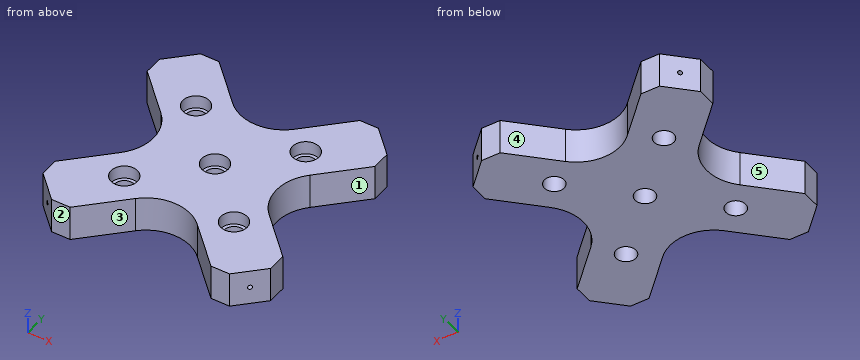
```python
from build123d import *

# Parameters (mm, degrees)
ESQUISSE1_R               = 2.25
BOSS_EXTRU_1_DEPTH        = 8
CONG_1_R                  = 10
ESQUISSE2_R               = 0.5
ENL_V_MAT_EXTRU_1_DEPTH   = 10
ESQUISSE3_R               = 3
ENL_V_MAT_EXTRU_2_DEPTH   = 3
SYM_TRIE2_COPY_1_SKETCH_R = 0.5
SYM_TRIE2_COPY_1_DEPTH    = 10
SYM_TRIE2_COPY_2_SKETCH_R = 3
SYM_TRIE2_COPY_2_DEPTH    = 3


with BuildPart() as part:
    # Esquisse1 → Boss.-Extru.1 (new body)
    with BuildSketch(Plane.XY):
        Polygon((-9.899494937, 0), (-25.935028843, 16.035533906), (-25.935028843, 20.278174593), (-20.278174593, 25.935028843), (-16.035533906, 25.935028843), (0, 9.899494937), (16.035533906, 25.935028843), (20.278174593, 25.935028843), (25.935028843, 20.278174593), (25.935028843, 16.035533906), (9.899494937, 0), (25.935028843, -16.035533906), (25.935028843, -20.278174593), (20.278174593, -25.935028843), (16.035533906, -25.935028843), (0, -9.899494937), (-16.035533906, -25.935028843), (-20.278174593, -25.935028843), (-25.935028843, -20.278174593), (-25.935028843, -16.035533906), align=None)
        with Locations((-12.5, -12.5)):
            Circle(ESQUISSE1_R, mode=Mode.SUBTRACT)
        with Locations((12.5, -12.5)):
            Circle(ESQUISSE1_R, mode=Mode.SUBTRACT)
        Circle(ESQUISSE1_R, mode=Mode.SUBTRACT)
        with Locations((12.5, 12.5)):
            Circle(ESQUISSE1_R, mode=Mode.SUBTRACT)
        with Locations((-12.5, 12.5)):
            Circle(ESQUISSE1_R, mode=Mode.SUBTRACT)
    extrude(amount=BOSS_EXTRU_1_DEPTH)

    # Congé1
    cong_1_edges = [part.edges().sort_by_distance(p)[0] for p in [
        (0, 9.899494937, 4),
        (9.899494937, 0, 4),
        (0, -9.899494937, 4),
        (-9.899494937, 0, 4),
    ]]
    fillet(cong_1_edges, radius=CONG_1_R)

    # Esquisse2 → Enlèv. mat.-Extru.1 (cut)
    with BuildSketch(Plane(origin=(23.106601718, 23.106601718, 0), x_dir=(0, 0, -1), z_dir=(0.707106781, 0.707106781, 0))):
        with Locations((-4, 0)):
            Circle(ESQUISSE2_R)
    enl_v_mat_extru_1 = extrude(amount=-ENL_V_MAT_EXTRU_1_DEPTH, mode=Mode.SUBTRACT)

    # Esquisse3 → Enlèv. mat.-Extru.2 (cut)
    with BuildSketch(Plane.XY.offset(8)):
        with Locations((12.5, 12.5)):
            Circle(ESQUISSE3_R)
        Circle(ESQUISSE3_R)
    enl_v_mat_extru_2 = extrude(amount=-ENL_V_MAT_EXTRU_2_DEPTH, mode=Mode.SUBTRACT)

    # Symétrie1: Enlèv. mat.-Extru.1, Enlèv. mat.-Extru.2 across plane
    add(enl_v_mat_extru_1.mirror(Plane.ZX), mode=Mode.SUBTRACT)
    add(enl_v_mat_extru_2.mirror(Plane.ZX), mode=Mode.SUBTRACT)

    # Symétrie2: Enlèv. mat.-Extru.1, Enlèv. mat.-Extru.2 across plane
    add(enl_v_mat_extru_1.mirror(Plane(origin=(0, 0, 0), x_dir=(0, 0, 1), z_dir=(1, 0, 0))), mode=Mode.SUBTRACT)
    add(enl_v_mat_extru_2.mirror(Plane(origin=(0, 0, 0), x_dir=(0, 0, 1), z_dir=(1, 0, 0))), mode=Mode.SUBTRACT)

    # Symétrie2 copy 1 sketch → Symétrie2 copy 1 (cut)
    with BuildSketch(Plane(origin=(-23.106601718, -23.106601718, 0), x_dir=(0, 0, -1), z_dir=(-0.707106781, -0.707106781, 0))):
        with Locations((-4, 0)):
            Circle(SYM_TRIE2_COPY_1_SKETCH_R)
    extrude(amount=-SYM_TRIE2_COPY_1_DEPTH, mode=Mode.SUBTRACT)

    # Symétrie2 copy 2 sketch → Symétrie2 copy 2 (cut)
    with BuildSketch(Plane(origin=(0, 0, 8), x_dir=(-1, 0, 0), z_dir=(0, 0, 1))):
        with Locations((12.5, 12.5)):
            Circle(SYM_TRIE2_COPY_2_SKETCH_R)
        Circle(SYM_TRIE2_COPY_2_SKETCH_R)
    extrude(amount=-SYM_TRIE2_COPY_2_DEPTH, mode=Mode.SUBTRACT)


solid = part.part
```
Geometry check sheet. Reference: the model listing, model coordinates, mm. Face numbers are marked on the shaded views. A direction names the side the tool comes from. Coordinates: 2 decimals unless noted, no trailing zeros. Write each loop counter-clockwise with the first axis right and the second up, starting at its lowest first coordinate (ties: lowest second). Pieces come first, ordered by that corner, then holes. Notation, with made-up numbers: M 11.5,-20 L 47.5,-20 A16 ccw 47.5,-15 Z; hole C -10,48.5 d1. An arc over 180 degrees is marked long. One line per item, written item: value. Start each with the question number.
(1) Sectioned sample at C-C, the plane y = 12.5. Enter the section's corners in (x, z).
(2) Scan lines: line 1 along X through (y, z) = (-11, 3.5); line 2 along Y through (x, z) = (16, 4); line 3 along Y through (x, z) = (-19, 3.75). Record each from-to range of solid material in increasing order. Write a range as [from, to].
(3) Sectioned sample at A-A, the plane x = 0. Enter the section's corners in (y, z).
(4) Depth check by flat-ended pin: pin 1 (3 mm diameter, centred on y = 15, z = 7, fed in from +X) (3 decimals); pin 2 (4 mm diameter, centred on x = 11.5, z = 1.5, fed in from +Y); pin 3 (5 mm diameter, centred on x = 0, y = 0, fed in from +Z). Enter the tip coordinate at first touch or a pass-through.
(5) Sectioned sample at B-B, the plane z = 6. State how many separate pieces and enclosed holes the cut face has, and give its area (3 significant figures).
(6) Release check for a two-part mould opening along Y. For the marked faces 3, 4 and 5 record: released by +Y, released by -Y, zero draft, split by the parting line, or undercut.
(7) Tool access check on the marked faces 1 and 2. Record the directions out of +Z, -Z, +X, -X, +Y, -Y that give a thin tool (end or side, any length) a straight path to the whole face; none if there is none.
Filled sheet:
1. outline: M -22.4,0 L -14.75,0 L -14.75,5 L -15.5,5 L -15.5,8 L -22.4,8 Z; M -10.25,0 L 10.25,0 L 10.25,5 L 9.5,5 L 9.5,8 L -9.5,8 L -9.5,5 L -10.25,5 Z; M 14.75,0 L 22.4,0 L 22.4,8 L 15.5,8 L 15.5,5 L 14.75,5 Z
2. line 1: [-20.9, -14.18], [-10.82, 10.82], [14.18, 20.9]
2. line 2: [-25.9, -16.71], [-16.07, -5.94], [5.94, 16.07], [16.71, 25.9]
2. line 3: [-25.94, -19.61], [-18.39, -9.1], [9.1, 18.39], [19.61, 25.94]
3. outline: M -14.04,0 L -2.25,0 L -2.25,5 L -3,5 L -3,8 L -14.04,8 Z; M 2.25,0 L 14.04,0 L 14.04,8 L 3,8 L 3,5 L 2.25,5 Z
4. pin 1: x = 25.935
4. pin 2: y = 23.4
4. pin 3: z = 5
5. separate pieces: 1
5. enclosed holes: 5
5. area: 1,540 mm²
6. face 3: released by -Y
6. face 4: released by +Y
6. face 5: undercut
7. face 1: +Z, -Z, +X
7. face 2: +Z, -Z, +X, -X, -Y
